Geometry: see drawing. Coordinates: mm, zero at the bounding-box minimum. Coordinates: 2 decimals unless noted, no trailing zeros. Order: outer loops, then holes, each group sorted by start corner. A loop starts at its lowest first (then second) coordinate and runs counter-clockwise, first axis right, second up.
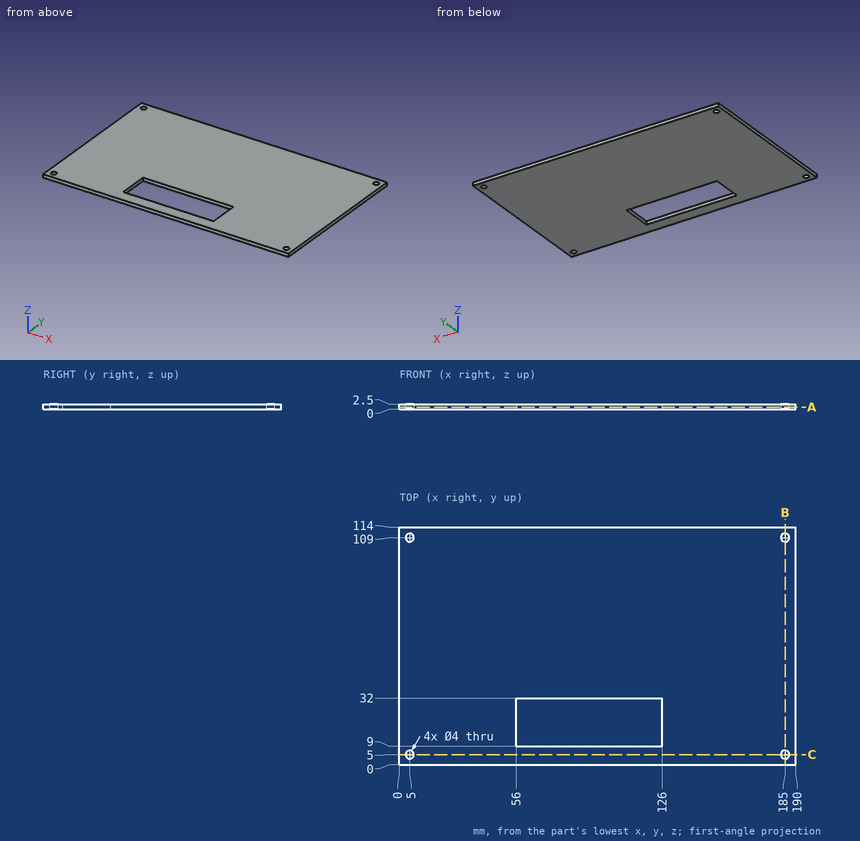
Item 1: Cut plane B-B on x = 185. Return loops of the section in (y, z).
Response values:
outline: (0, 0) - (3, 0) - (3, 2.5) - (0, 2.5) - close; (7, 0) - (107, 0) - (107, 2.5) - (7, 2.5) - close; (111, 0) - (114, 0) - (114, 2.5) - (111, 2.5) - close
Item 2: Cut plane A-A on z = 0.95. Return loops of the section in (x, y).
Response values:
outline: (0, 0) - (190, 0) - (190, 114) - (0, 114) - close; hole circle Ø4 at (5, 5); hole circle Ø4 at (5, 109); hole (56, 9) - (126, 9) - (126, 32) - (56, 32) - close; hole circle Ø4 at (185, 5); hole circle Ø4 at (185, 109)
Item 3: Cut plane C-C on y = 5. Return loops of the section in (x, z).
Response values:
outline: (0, 0) - (3, 0) - (3, 2.5) - (0, 2.5) - close; (7, 0) - (183, 0) - (183, 2.5) - (7, 2.5) - close; (187, 0) - (190, 0) - (190, 2.5) - (187, 2.5) - close
Item 4: Ray query, probe 1 along Y at (x, z) = (5, 1.2); probe 2 along X at (y, z) = (109, 0.7); probe 3 along X at (y, z) = (28, 0.5). Return the intervals inside material, ascending.
Response values:
probe 1: y = 0 to 3, 7 to 107, 111 to 114
probe 2: x = 0 to 3, 7 to 183, 187 to 190
probe 3: x = 0 to 56, 126 to 190
